Could you check a few things on this model? Use its own coordinates, in mm. A direction names the side the tool comes from. Round coordinates to 2 decimals unless told otherwise and drop trailing zeros. Loops run counter-clockwise (first coordinate to the right, second up) from the corner with the lowest first, then second, coordinate; pieces in that order, holes last. Notation, with made-up numbers: M 64.25,14.25 L 113.25,14.25 A29 ccw 113.25,46.25 Z; hole C 36.5,34 d11. An arc over 180 degrees is marked long. Answer in a Markdown table with one row per item.
```python
from build123d import *

# Parameters (mm, degrees)
F0_W         = 12
F0_H         = 10
F1_DEPTH     = 14
F2_R         = 2.25
F3_DEPTH     = 99.1
F4_DEPTH     = 25
F5_R         = 6.2769552622
F6_R         = 6.2769552622
F7_R         = 2.5
F8_R         = 2.5
F9_R         = 2.5
F10_R        = 2.5
F11_T1_DEPTH = 14
F11_T3_DEPTH = 21.0473321416
F11_T5_DEPTH = 26.9573104187
F12_R        = 7.2
F13_R        = 7.2
F14_R        = 0.5445837107


# Not quite as in the source:
# - a fillet or chamfer that OpenCascade refuses, or shapes differently, is made with other operations: its cross-section is extruded or revolved along the edge and cut away or added


with BuildPart() as f1:
    # F0 (on Front) → F1 (new body)
    with BuildSketch(Plane.XZ):
        Polygon((59.6290528774, 0), (74.6290528774, 0), (74.6890899837, 3.3114668612), (59.6890899837, 3.3114668612), (59.6890899837, 14.3114668612), (74.6890899837, 14.3114668612), (74.6890899837, 24.3114668612), (47.2866145434, 24.3114668612), (34.3200196198, 19.0325071069), (5.3200196198, 19.0325071069), (-4.6910188856, 27.3114668612), (-17.6799803802, 27.3114668612), (-17.6799803802, 24.3114668612), (-4.6910188856, 24.3114668612), (1.3200196198, 19.0325071069), (-17.6799803802, 19.0325071069), (-17.6799803802, 16.0325071069), (5.3200196198, 16.0325071069), (5.3200196198, 6.0325071069), (-17.6799803802, 6.0325071069), (-17.6799803802, 3.0325071069), (53.3200196198, 3.0325071069), align=None)
        with Locations((13.8200196198, 11.0325071069)):
            Rectangle(F0_W, F0_H, mode=Mode.SUBTRACT)
        with Locations((28.3200196198, 11.0325071069)):
            Rectangle(F0_W, F0_H, mode=Mode.SUBTRACT)
        Polygon((55.8200196198, 6.0325071069), (36.8200196198, 6.0325071069), (36.8200196198, 14.8739311844), (47.7449782193, 19.0325071069), (55.8200196198, 19.0325071069), align=None, mode=Mode.SUBTRACT)
    extrude(amount=F1_DEPTH)

    # F2 (on Top) → F3 (cut)
    with BuildSketch(Plane.XY):
        with Locations((-9.0681398287, -7.2300466709)):
            Circle(F2_R)
        with Locations((67.4190670252, -7.2234715335)):
            Circle(F2_R)
    extrude(amount=F3_DEPTH, mode=Mode.SUBTRACT)

    # F2 (on Top) → F4 (cut)
    with BuildSketch(Plane.XY):
        with Locations((-9.0681398287, -7.2300466709)):
            Circle(F2_R)
        with Locations((67.4190670252, -7.2234715335)):
            Circle(F2_R)
    extrude(amount=-F4_DEPTH, mode=Mode.SUBTRACT)

    # F5
    f5_edges = [f1.edges().sort_by_distance(p)[0] for p in [
        (-17.67998, -14, 25.811467),
        (-17.67998, 0, 25.811467),
        (-17.67998, -14, 17.532507),
        (-17.67998, 0, 17.532507),
        (-17.67998, 0, 4.532507),
        (-17.67998, -14, 4.532507),
    ]]
    fillet(f5_edges, radius=F5_R)

    # F6
    f6_edges = [f1.edges().sort_by_distance(p)[0] for p in [
        (74.68909, -14, 19.311467),
        (74.68909, 0, 19.311467),
        (74.659071, -14, 1.655733),
        (74.659071, 0, 1.655733),
    ]]
    fillet(f6_edges, radius=F6_R)

    # F7
    f7_edges = [f1.edges().sort_by_distance(p)[0] for p in [
        (36.82002, -7, 6.032507),
        (36.82002, -7, 14.873931),
        (47.744978, -7, 19.032507),
        (55.82002, -7, 19.032507),
        (55.82002, -7, 6.032507),
    ]]
    fillet(f7_edges, radius=F7_R)

    # F8
    f8_edges = [f1.edges().sort_by_distance(p)[0] for p in [
        (34.32002, -7, 16.032507),
        (22.32002, -7, 16.032507),
        (22.32002, -7, 6.032507),
        (34.32002, -7, 6.032507),
    ]]
    fillet(f8_edges, radius=F8_R)

    # F9
    f9_edges = [f1.edges().sort_by_distance(p)[0] for p in [
        (19.82002, -7, 16.032507),
        (7.82002, -7, 16.032507),
        (7.82002, -7, 6.032507),
        (19.82002, -7, 6.032507),
    ]]
    fillet(f9_edges, radius=F9_R)

    # F10
    f10_edges = [f1.edges().sort_by_distance(p)[0] for p in [
        (5.32002, -7, 16.032507),
        (5.32002, -7, 6.032507),
        (59.68909, -7, 14.311467),
        (59.68909, -7, 3.311467),
    ]]
    fillet(f10_edges, radius=F10_R)

    # F11: fillet of radius 7.2 on 4 edges, made by hand

    # F11_s2 → F11_t1 (join)
    with BuildSketch(Plane.XZ):
        with BuildLine():
            ThreePointArc((35.6254467793, 19.5639725748), (34.2937652809, 19.1666225681), (32.9105531914, 19.0325071069))
            Line((32.9105531914, 19.0325071069), (34.3200196198, 19.0325071069))
            Line((34.3200196198, 19.0325071069), (35.6254467793, 19.5639725748))
        make_face()
        with BuildLine():
            ThreePointArc((7.9114817035, 19.0325071069), (5.4731495991, 19.457956454), (3.3229804953, 20.6840247322))
            Line((3.3229804953, 20.6840247322), (5.3200196198, 19.0325071069))
            Line((5.3200196198, 19.0325071069), (7.9114817035, 19.0325071069))
        make_face()
    extrude(amount=F11_T1_DEPTH)

    # F11_s4 → F11_t3 (cut)
    with BuildSketch(Plane.XZ.offset(-3.5236660708)):
        with BuildLine():
            ThreePointArc((48.6960809717, 24.3114668612), (47.3128688823, 24.1773514), (45.9811873838, 23.7800013933))
            Line((45.9811873838, 23.7800013933), (47.2866145434, 24.3114668612))
            Line((47.2866145434, 24.3114668612), (48.6960809717, 24.3114668612))
        make_face()
    extrude(amount=F11_T3_DEPTH, mode=Mode.SUBTRACT)

    # F11_s6 → F11_t5 (cut)
    with BuildSketch(Plane.XZ.offset(-6.4786552093)):
        with BuildLine():
            ThreePointArc((-2.6939797611, 25.6599492359), (-4.844148865, 26.8860175141), (-7.2824809693, 27.3114668612))
            Line((-7.2824809693, 27.3114668612), (-4.6910188856, 27.3114668612))
            Line((-4.6910188856, 27.3114668612), (-2.6939797611, 25.6599492359))
        make_face()
    extrude(amount=F11_T5_DEPTH, mode=Mode.SUBTRACT)

    # F12
    f12_edges = [f1.edges().sort_by_distance(p)[0] for p in [
        (53.32002, -7, 3.032507),
        (59.629053, -7, 0),
    ]]
    fillet(f12_edges, radius=F12_R)

    # F13
    f13_edges = [f1.edges().sort_by_distance(p)[0] for p in [
        (-4.691019, -7, 24.311467),
    ]]
    fillet(f13_edges, radius=F13_R)

    # F14
    f14_edges = [f1.edges().sort_by_distance(p)[0] for p in [
        (1.32002, -7, 19.032507),
    ]]
    fillet(f14_edges, radius=F14_R)


solid = f1.part
```
1) I want a section at B-B, the plane y = -3. State how many separate pieces and enclosed holes the cut face has, plus the area to 3 significant figures.
Computed:
| item | result |
|---|---|
| separate pieces | 1 |
| enclosed holes | 3 |
| area | 919 mm² |
2) If we mould it in two halves opening along Z, with no side actions, what happens to faces 1 (the face through (56.45, -6.9, 1.53)), 2 (the face through (23.072, -7.098, 6.745)), 3 (the face through (40.876, -6.902, 21.701))? For each: released by +Z, released by -Z, zero draft, split by the parting line, or undercut.
Computed:
| item | result |
|---|---|
| face 1 | released by -Z |
| face 2 | undercut |
| face 3 | released by +Z |
3) I want a section at A-A, the plane x = 44.5. Please give me the cut outline in (y, z).
Computed:
| item | result |
|---|---|
| outline | M -14,3.03 L 0,3.03 L 0,6.03 L -14,6.03 Z; M -14,17.8 L 0,17.8 L 0,23.18 L -14,23.18 Z |
4) I need wall thicknesses on line 1 (X direction, y = -4.5, z = 9); line 2 (Z direction, x = -7.5, y = -13); line 3 (Z direction, x = 11, y = -6.75). Which ranges of each line are inside material? Lowest first, please.
Computed:
| item | result |
|---|---|
| line 1 | x = 5.32 to 7.82, 19.82 to 22.32, 34.32 to 36.82, 55.82 to 59.69 |
| line 2 | z = 3.03 to 6.03, 16.03 to 19.03, 24.31 to 27.31 |
| line 3 | z = 3.03 to 6.03, 16.03 to 19.03 |
5) Which directions (+Z, -Z, +X, -X, +Y, -Y) give clear straight access to the entire face, cutting with the end or side of a thin tool? Please do faces 4 (the face through (17, -7, 3.033)), 5 (the face through (5.32, -7, 11)), 6 (the face through (34.32, -7, 11)).
Computed:
| item | result |
|---|---|
| face 4 | -Z, -X, +Y, -Y |
| face 5 | -X, +Y, -Y |
| face 6 | +Y, -Y |
6) Will these pins go through, and if not, where does the flat tip stop? P1, Ø6, axis at x = 64, y = -6, coming from the +Z side; P2, Ø1.5, axis at y = -3.5, z = 11, coming from the +X side; P3, Ø2, axis at x = 27.5, y = -4, coming from the +Z side; P4, Ø2, axis at x = -3, z = 9, coming from the -Y side.
Computed:
| item | result |
|---|---|
| P1 | stops at z = 24.31 |
| P2 | stops at x = 59.69 |
| P3 | stops at z = 19.03 |
| P4 | passes through |
